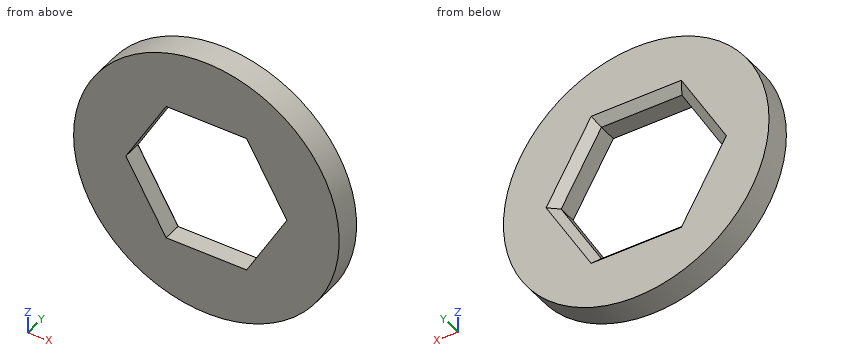
Autodesk Inventor part; units mm, degrees
ref_plane "YZ Plane" through (0, 0, 0) normal (1, 0, 0) x (0, 1, 0)
ref_plane "XZ Plane" through (0, 0, 0) normal (0, 1, 0) x (-1, 0, 0)
ref_plane "XY Plane" through (0, 0, 0) normal (0, 0, 1) x (1, 0, 0)
sketch "Sketch9" plane through (0, 0, 0) normal (0, 1, 0) x (-1, 0, 0)
  circle A0 centre (0, 0) radius 12.6365
  dimension "d53" = 25.273
extrude "Extrusion6" add sketch "Sketch9" along normal mid plane 2.54
sketch "Sketch15" plane through (0, 1.27, 0) normal (0, 1, 0) x (1, 0, 0)
  line L0 (7.6623, 0) -> (3.8312, -6.6357)
  line L1 (3.8312, -6.6357) -> (-3.8312, -6.6357)
  line L2 (-3.8312, -6.6357) -> (-7.6623, 0)
  line L3 (-7.6623, 0) -> (-3.8312, 6.6357)
  line L4 (-3.8312, 6.6357) -> (3.8312, 6.6358)
  line L5 (3.8312, 6.6358) -> (7.6623, 0)
  point P0 (0, 0)
  point P1 (0, 0)
  dimension "d82" = 13.2715
extrude "Extrusion11" cut sketch "Sketch15" against normal through all
chamfer "Chamfer7" distance 0.7937 angle 45 6 edges at (-5.7467, 1.27, -3.3179) (-5.7467, 1.27, 3.3179) (0, 1.27, 6.6357) (5.7467, 1.27, 3.3179) (5.7467, 1.27, -3.3179) (0, 1.27, -6.6358)
equation "\"d82\" = hexDiameter"
equation "\"holeForString\" = stringDiameter + clearanceForString"
equation "\"stringDiameter\" = 3.048"
equation "\"clearanceForString\" = 2.032"
equation "\"spoolHeightWithoutSpacer\" = 69.85"
equation "\"hexShaftDiameter\" = 12.7"
equation "\"clearanceForHexShaft\" = 0.5715"
equation "\"hexDiameter\" = hexShaftDiameter + clearanceForHexShaft"
equation "\"supportChannels\" = 3.81"
equation "\"spoolInteriorDiameter\" = 38.1"
equation "\"spoolInteriroRadius\" = 0.5 * spoolInteriorDiameter"
equation "\"spoolExteriorDiameter\" = 88.9"
equation "\"spoolExteriorRadius\" = 0.5 * spoolExteriorDiameter"
equation "\"spoolFiletRadius\" = 0.5 * supportChannels"
equation "\"holeCenter\" = 0.25 * spoolHeightWithoutSpacer - 0.75 * supportChannels"
equation "\"hexHoleChamfer\" = 1.5875"
equation "\"stringHoleCenterFromHexShaft\" = 0.5 * hexDiameter + 0.5 * holeForString"
equation "\"textCircleDiameter\" = 0.75 * spoolExteriorDiameter"
equation "\"textHeight\" = 6.096"
equation "\"textDepth\" = 1.27"
equation "\"stringHoleChamfer\" = 4.7625"
equation "\"spoolTotalHeight\" = 76.2"
equation "\"spaceHeight\" = spoolTotalHeight - spoolHeightWithoutSpacer"
equation "\"spacerDiameter\" = 24.13"
properties part number "spacerForEndV05" material "PC/ABS Plastic"
Here's how the part is built. I have some questions about the finished solid (model axes, mm). Coordinates: 2 decimals unless noted, no trailing zeros. Loops run counter-clockwise (first coordinate to the right, second up) from the corner with the lowest first, then second, coordinate; pieces in that order, holes last. Notation, with made-up numbers: (-32, -9.5) -> (-18, -9.5) arc R27 cw to (-18, 25.5) -> close; hole circle Ø9 at (30.25, 60.25). An arc over 180 degrees is marked (long way). Use one line per item in the form item = value. Start each with the question number.
(1) If we section it at D-D (z = 10.25): Please give me the cut outline in (x, y).
(2) Please list where these lines run through material, in increasing order: line 1 along Z through (x, y) = (0.75, -0.55); line 2 along X through (y, z) = (0.5, 1.5); line 3 along Z through (x, y) = (6.75, 0.55).
(3) If we section it at A-A (y = -0.05): Please give me the cut outline in (x, z), then the cut area to 3 significant figures.
(4) Will these pins go through, and if not, where does the flat tip stop? pin 1 (1 mm diameter, centred on y = -0.5, z = 4.5, fed in from +X); pin 2 (0.5 mm diameter, centred on x = 1, y = 0, fed in from +Z); pin 3 (0.9 mm diameter, centred on x = 1, y = 0, fed in from -Z).
(5) If we section it at B-B (x = -0.5): Please give me the cut outline in (y, z), then the cut area to 3 significant figures.
(6) If we section it at C-C (z = -3.25): Please give me the cut outline in (x, y).
Verdict:
q1.outline = (-7.39, -1.27) -> (7.39, -1.27) -> (7.39, 1.27) -> (-7.39, 1.27) -> close
q2.line_1 = -12.61 to -6.64, 6.64 to 12.61
q2.line_2 = -12.55 to -6.82, 6.82 to 12.55
q2.line_3 = -10.68 to -1.73, 1.73 to 10.68
q3.outline = circle Ø25.27 at (0, 0); hole (-7.66, 0) -> (-3.83, -6.64) -> (3.83, -6.64) -> (7.66, 0) -> (3.83, 6.64) -> (-3.83, 6.64) -> close
q3.area = 349 mm²
q4.pin_1 = 11.99
q4.pin_2 = 12.61
q4.pin_3 = -12.62
q5.outline = (-1.27, -12.63) -> (1.27, -12.63) -> (1.27, -7.43) -> (0.48, -6.64) -> (-1.27, -6.64) -> close; (-1.27, 6.64) -> (0.48, 6.64) -> (1.27, 7.43) -> (1.27, 12.63) -> (-1.27, 12.63) -> close
q5.area = 29.8 mm²
q6.outline = (-12.21, -1.27) -> (-5.79, -1.27) -> (-5.79, 0.48) -> (-6.7, 1.27) -> (-12.21, 1.27) -> close; (5.79, -1.27) -> (12.21, -1.27) -> (12.21, 1.27) -> (6.7, 1.27) -> (5.79, 0.48) -> close
